Drawing for the job (mm, zero at the part's lowest x, y, z). Coordinates: 2 decimals unless noted, no trailing zeros. Loops run counter-clockwise (first coordinate to the right, second up) from the corner with the lowest first, then second, coordinate; pieces in that order, holes last. Notation, with made-up numbers: (9.25, -17) -> (19.25, -17) arc R28 ccw to (19.25, 7) -> close; hole circle Ø5 at (-11.5, -32.5). An arc over 180 degrees is marked (long way). Write each question's results on one line, items separated by ' | '.
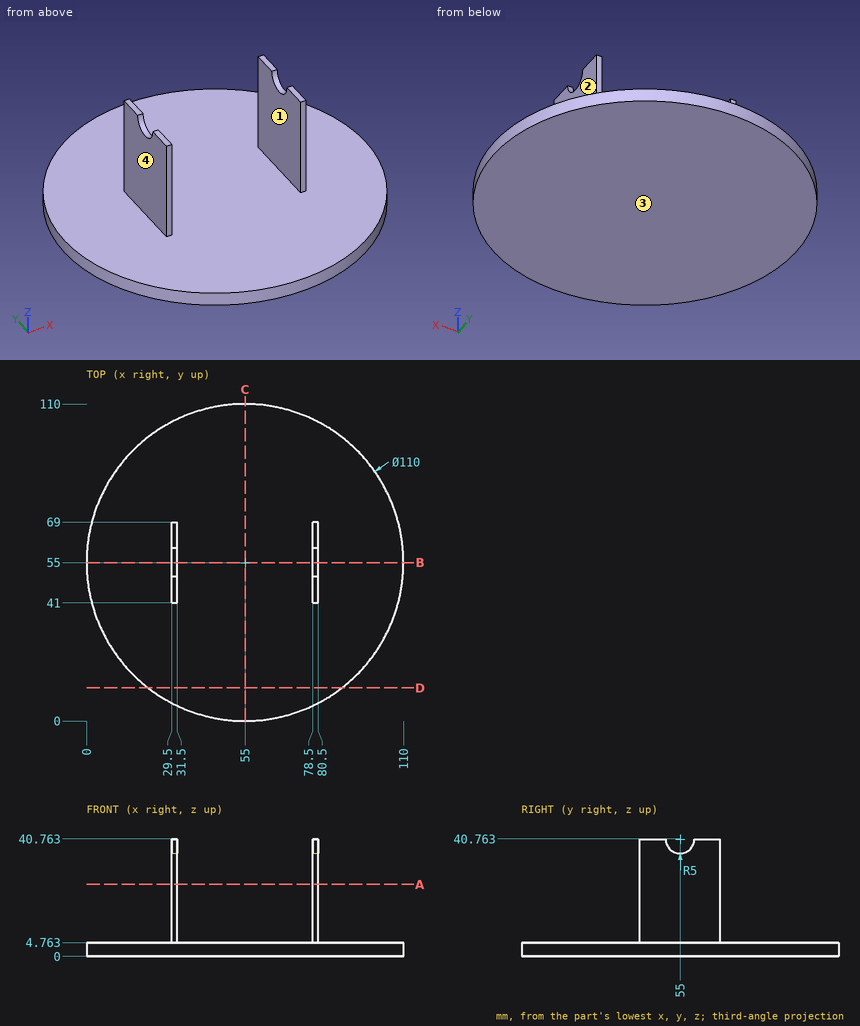
1) Slice it at C-C (x = 55). Write the cut outline in (y, z).
Outcome:
outline: (0, 0) -> (110, 0) -> (110, 4.76) -> (0, 4.76) -> close
2) Slice it at B-B (y = 55). Write the cut outline in (x, z), then the cut area to 3 significant figures.
Outcome:
outline: (0, 0) -> (110, 0) -> (110, 4.76) -> (80.5, 4.76) -> (80.5, 35.76) -> (78.5, 35.76) -> (78.5, 4.76) -> (31.5, 4.76) -> (31.5, 35.76) -> (29.5, 35.76) -> (29.5, 4.76) -> (0, 4.76) -> close | area: 648 mm^2
3) Pin check, flat tips, straight feed: pin 1 (0.6 mm diameter, centred on x = 80, z = 29, fed in from -Y); pin 2 (2 mm diameter, centred on x = 80, z = 27.5, fed in from +Y); pin 3 (22.5 mm diameter, centred on y = 61.5, z = 25.5, fed in from -X). Stop position of each tip, or through.
Outcome:
pin 1: stops at y = 41 | pin 2: stops at y = 69 | pin 3: stops at x = 29.5
4) Slice it at D-D (y = 11.5). Write the cut outline in (x, z).
Outcome:
outline: (21.34, 0) -> (88.66, 0) -> (88.66, 4.76) -> (21.34, 4.76) -> close
5) Drill centre lines: L1, parallel to X at y = 61, z = 34.5; L2, parallel to Z at x = 70, y = 85; L3, parallel to X at y = 88, z = 2.5. Where is each one in solid material? Low to high. Write a range as from..to.
Outcome:
L1: x = 29.5..31.5, 78.5..80.5 | L2: z = 0..4.76 | L3: x = 11..99
6) Slice it at A-A (z = 25). Write the cut outline in (x, y).
Outcome:
outline: (29.5, 41) -> (31.5, 41) -> (31.5, 69) -> (29.5, 69) -> close; (78.5, 41) -> (80.5, 41) -> (80.5, 69) -> (78.5, 69) -> close
7) Two-plate mould, pull along X, no slides. Class the marked faces 1, 2, 3 and 4: pulls with the +X half, pulls with the -X half, needs draft (parallel to the pull), parting line crosses it, or undercut.
Outcome:
face 1: undercut | face 2: pulls with the +X half | face 3: needs draft | face 4: pulls with the -X half
